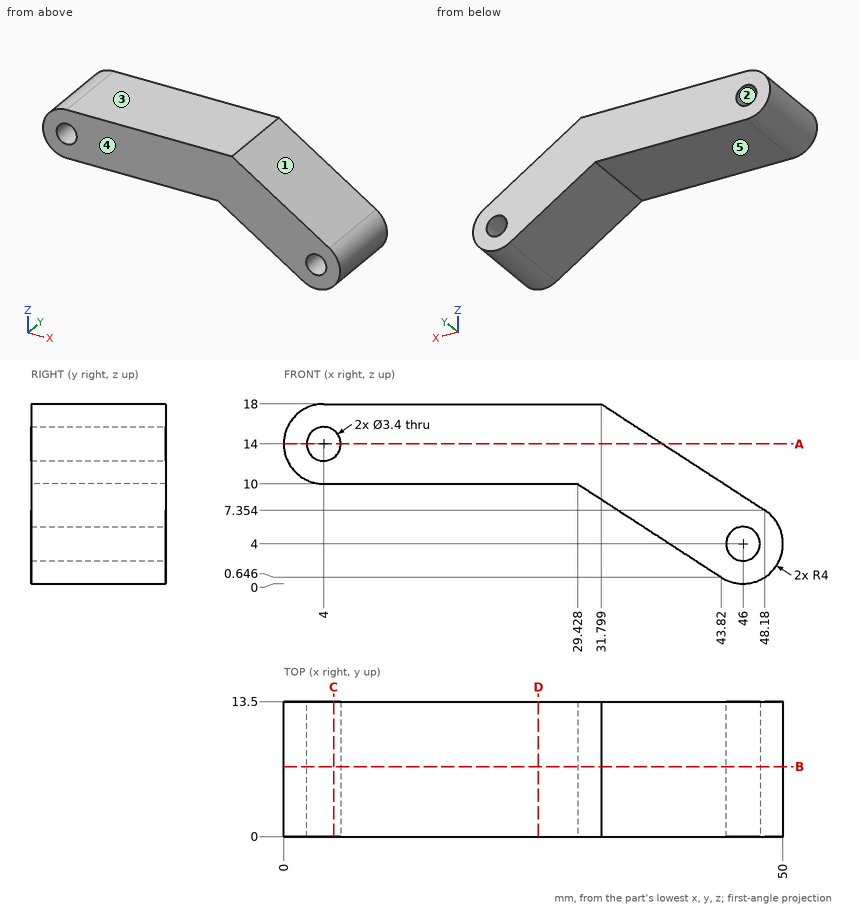
The drawing under review shows one solid part. Ordinate dimensions are in mm from its lowest x, y, z. A direction names the side the tool comes from. Round coordinates to 2 decimals unless told otherwise and drop trailing zeros. Loops run counter-clockwise (first coordinate to the right, second up) from the corner with the lowest first, then second, coordinate; pieces in that order, holes last.
Item 1: Mouldability with a two-part tool opening along X and no side actions: class the marked faces 1, 2 and 3 as released by +X, released by -X, zero draft, split by the parting line, or undercut.
Determined:
face 1: released by +X
face 2: undercut
face 3: zero draft
Item 2: Take a section at A-A (z = 14). Write out the cut boundary in (x, y).
Determined:
outline: (0, 0) - (2.3, 0) - (2.3, 13.5) - (0, 13.5) - close; (5.7, 0) - (37.95, 0) - (37.95, 13.5) - (5.7, 13.5) - close
Item 3: Take a section at B-B (y = 7). Write out the cut boundary in (x, z).
Determined:
outline: (4, 10) - (29.43, 10) - (43.82, 0.65) arc R4 ccw to (48.18, 7.35) - (31.8, 18) - (4, 18) arc R4 ccw to start; hole circle Ø3.4 at (4, 14); hole circle Ø3.4 at (46, 4)
Item 4: Clearance check with flat-ended pins moving along their axes: pin 1 Ø1 at (x, y) = (44.5, 1.5) entering from -Z; pin 2 Ø4 at (x, y) = (19.5, 3.5) entering from -Z; pin 3 Ø6 at (y, z) = (10, 10.5) entering from +X (1 decimal). State where each tip first meets the part, or that it passes through.
Determined:
pin 1: stops at z = 0.13
pin 2: stops at z = 10
pin 3: stops at x = 48
Item 5: Take a section at D-D (x = 25.5). Write out the cut boundary in (y, z), then the cut area to 3 significant figures.
Determined:
outline: (0, 10) - (13.5, 10) - (13.5, 18) - (0, 18) - close
area: 108 mm2
Item 6: For the marked faces 4 and 5, list the 3-axis set-ups (+Z, -Z, +X, -X, +Y, -Y) from which the entire face can be reached by the end or side of a thin tool; tool diameter is ignored.
Determined:
face 4: +Z, -Z, +X, -X, -Y
face 5: -Z, -X, +Y, -Y
Item 7: Take a section at C-C (x = 5). Write out the cut boundary in (y, z) (1 decimal).
Determined:
outline: (0, 10) - (13.5, 10) - (13.5, 12.6) - (0, 12.6) - close; (0, 15.4) - (13.5, 15.4) - (13.5, 18) - (0, 18) - close
Item 8: For line 1 (Z direction, x = 4, y = 9.25); line 2 (Z direction, x = 3, y = 9.5) (1 decimal); line 3 (Z direction, x = 22.5, y = 9), list the stretches that pass through material, from the lowest coordinate up.
Determined:
line 1: z = 10 to 12.3, 15.7 to 18
line 2: z = 10.1 to 12.6, 15.4 to 17.9
line 3: z = 10 to 18
